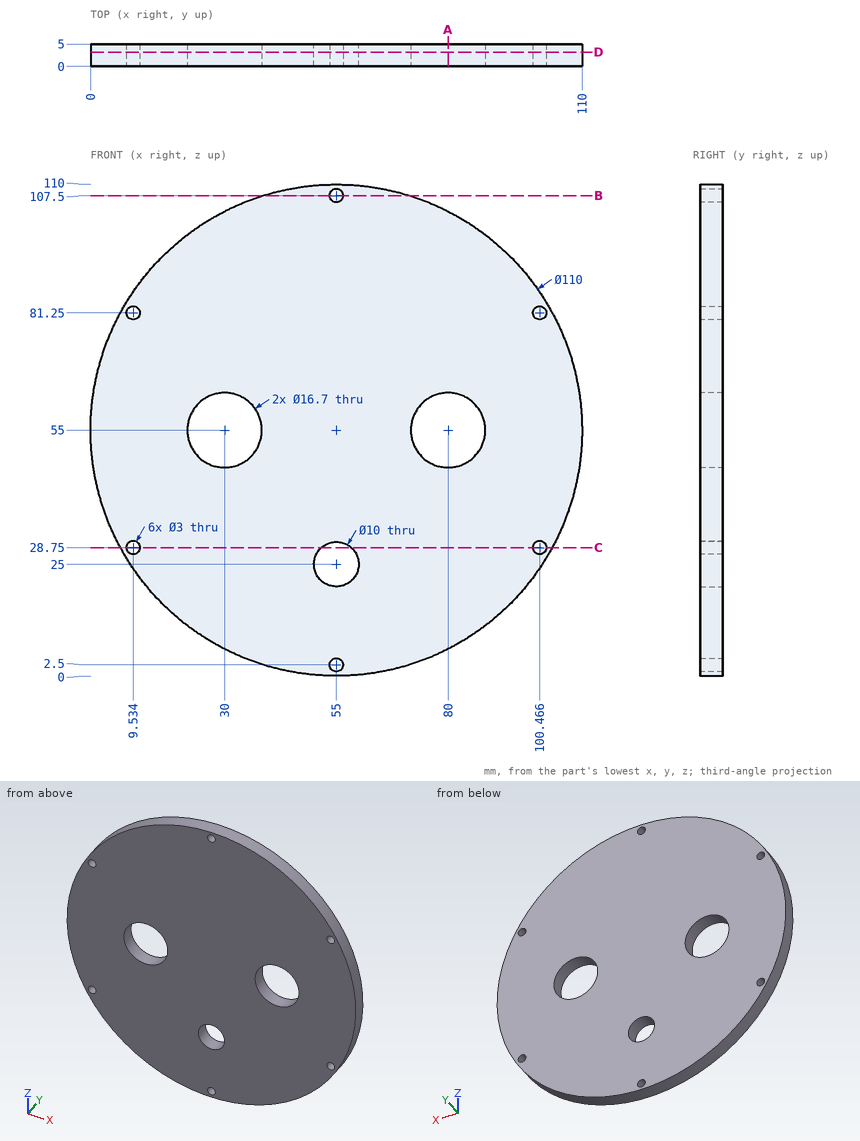
The figure shows three views and two pictorial views of one solid part (mm, origin at its lowest corner). Answer the questions. Coordinates: 2 decimals unless noted, no trailing zeros. Loops run counter-clockwise (first coordinate to the right, second up) from the corner with the lowest first, then second, coordinate; pieces in that order, holes last.
1) Find section C-C on z = 28.75. Write down the section's boundary in (x, y).
2) Find section B-B on z = 107.5. Write down the section's boundary in (x, y).
3) Flat-ended cylindrical pins translate along their axes: pin 1 Ø15 at (x, z) = (30, 55) entering from -Y; pin 2 Ø3.5 at (x, z) = (100.47, 28.75) entering from -Y; pin 3 Ø1 at (y, z) = (2.5, 84.5) entering from -X; pin 4 Ø3 at (x, y) = (68, 2) entering from +Z. Find the tip coordinate at first contact, or state that the pin passes through.
4) Find section D-D on y = 3.2. Give the number of separate pieces and of enclosed holes in the cut face, then the cut area to 3 significant figures.
5) Find the intervals of material crossed by L1, parallel to X at y = 1.9, z = 55; L2, parallel to Z at x = 101, y = 2.4; L3, parallel to X at y = 1.45, z = 81.25 (1 decimal), in increasing order.
6) Find section A-A on x = 80. Write down the section's boundary in (y, z).
Values:
1. outline: (6.67, 0) - (8.03, 0) - (8.03, 5) - (6.67, 5) - close; (11.03, 0) - (51.69, 0) - (51.69, 5) - (11.03, 5) - close; (58.31, 0) - (98.97, 0) - (98.97, 5) - (58.31, 5) - close; (101.97, 0) - (103.33, 0) - (103.33, 5) - (101.97, 5) - close
2. outline: (38.61, 0) - (53.5, 0) - (53.5, 5) - (38.61, 5) - close; (56.5, 0) - (71.39, 0) - (71.39, 5) - (56.5, 5) - close
3. pin 1: passes through
3. pin 2: stops at y = 0
3. pin 3: stops at x = 8.27
3. pin 4: stops at z = 108.78
4. separate pieces: 1
4. enclosed holes: 9
4. area: 8,940 mm2
5. L1: x = 0 to 21.65, 38.35 to 71.65, 88.35 to 110
5. L2: z = 24.85 to 27.35, 30.15 to 79.85, 82.65 to 85.15
5. L3: x = 6.7 to 8, 11 to 99, 102 to 103.3
6. outline: (0, 6.01) - (5, 6.01) - (5, 46.65) - (0, 46.65) - close; (0, 63.35) - (5, 63.35) - (5, 103.99) - (0, 103.99) - close
